The model under review builds one solid part; all positions refer to its coordinate system, in mm. Give positions to 0.01 mm unless a question says otherwise; leave off trailing zeros. Order: outer loops, then holes, each group sorted by start corner. A loop starts at its lowest first (then second) coordinate and runs counter-clockwise, first axis right, second up. Notation, with made-up numbers: (-2, -21.5) - (39, -21.5) arc R9 ccw to (39, -9.5) - close; hole circle Ø7 at (-39, 82). An arc over 180 degrees is marked (long way). Use CSV: the item, a comma, the result in double quotes. Start each with the question number.
```python
from build123d import *

# Parameters (mm, degrees)
SKETCH1_R           = 2.4892
BOSS_EXTRUDE1_DEPTH = 2.286


with BuildPart() as part:
    # Sketch1 → Boss-Extrude1 (new body)
    with BuildSketch(Plane.XY):
        with BuildLine():
            Line((459.749472964, 373.657281044), (426.729472964, 373.657281044))
            ThreePointArc((426.729472964, 373.657281044), (423.137370515, 375.145178596), (421.649472964, 378.737281044))
            Line((421.649472964, 378.737281044), (421.649472964, 387.627281044))
            ThreePointArc((421.649472964, 387.627281044), (423.137370515, 391.219383493), (426.729472964, 392.707281044))
            Line((426.729472964, 392.707281044), (537.219472964, 392.707281044))
            ThreePointArc((537.219472964, 392.707281044), (540.811575412, 391.219383493), (542.299472964, 387.627281044))
            Line((542.299472964, 387.627281044), (542.299472964, 277.137281044))
            ThreePointArc((542.299472964, 277.137281044), (540.811575412, 273.545178596), (537.219472964, 272.057281044))
            Line((537.219472964, 272.057281044), (528.329472964, 272.057281044))
            ThreePointArc((528.329472964, 272.057281044), (524.737370515, 273.545178596), (523.249472964, 277.137281044))
            Line((523.249472964, 277.137281044), (523.249472964, 310.157281044))
            ThreePointArc((523.249472964, 310.157281044), (504.650753569, 355.05856165), (459.749472964, 373.657281044))
        make_face()
        with Locations((431.174472964, 383.182281044)):
            Circle(SKETCH1_R, mode=Mode.SUBTRACT)
        with Locations((443.874472964, 383.182281044)):
            Circle(SKETCH1_R, mode=Mode.SUBTRACT)
        with Locations((456.574472964, 383.182281044)):
            Circle(SKETCH1_R, mode=Mode.SUBTRACT)
        with Locations((469.274472964, 383.182281044)):
            Circle(SKETCH1_R, mode=Mode.SUBTRACT)
        with Locations((481.974472964, 383.182281044)):
            Circle(SKETCH1_R, mode=Mode.SUBTRACT)
        with Locations((494.674472964, 383.182281044)):
            Circle(SKETCH1_R, mode=Mode.SUBTRACT)
        with Locations((507.374472964, 383.182281044)):
            Circle(SKETCH1_R, mode=Mode.SUBTRACT)
        with Locations((520.074472964, 383.182281044)):
            Circle(SKETCH1_R, mode=Mode.SUBTRACT)
        with Locations((532.774472964, 383.182281044)):
            Circle(SKETCH1_R, mode=Mode.SUBTRACT)
        with Locations((532.774472964, 370.482281044)):
            Circle(SKETCH1_R, mode=Mode.SUBTRACT)
        with Locations((532.774472964, 357.782281044)):
            Circle(SKETCH1_R, mode=Mode.SUBTRACT)
        with Locations((532.774472964, 345.082281044)):
            Circle(SKETCH1_R, mode=Mode.SUBTRACT)
        with Locations((532.774472964, 332.382281044)):
            Circle(SKETCH1_R, mode=Mode.SUBTRACT)
        with Locations((532.774472964, 319.682281044)):
            Circle(SKETCH1_R, mode=Mode.SUBTRACT)
        with Locations((532.774472964, 306.982281044)):
            Circle(SKETCH1_R, mode=Mode.SUBTRACT)
        with Locations((532.774472964, 294.282281044)):
            Circle(SKETCH1_R, mode=Mode.SUBTRACT)
        with Locations((532.774472964, 281.582281044)):
            Circle(SKETCH1_R, mode=Mode.SUBTRACT)
    extrude(amount=BOSS_EXTRUDE1_DEPTH)


solid = part.part
```
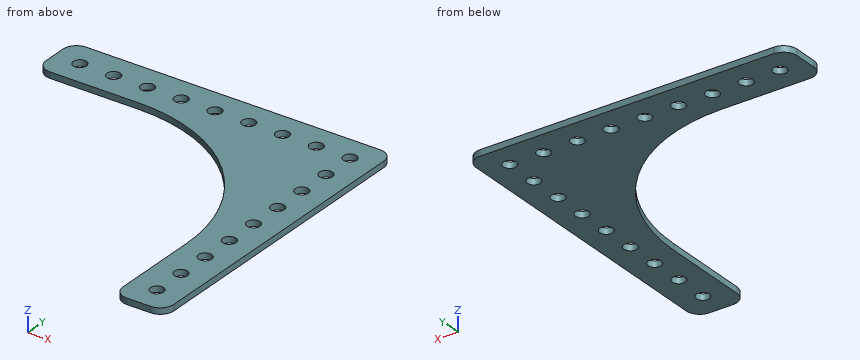
1. Consider section A-A (z = 1). State how many separate pieces and enclosed holes the cut face has, and give its area (3 significant figures).
2. Consider section B-B (x = 483). Give the boundary of the cut face in (y, z).
3. To check wall thickness, follow L1, parallel to X at y = 278, z = 1; L2, parallel to Y at x = 484, z = 1.7; L3, parallel to Y at x = 509, z = 2.15. State the ranges of each line that lie inside material, in increasing order. Write a range as [from, to].
4. Clearance check with flat-ended pins moving along their axes: pin 1 (6.5 mm diameter, centred on x = 532.77, y = 383.18, fed in from -Z); pin 2 (3 mm diameter, centred on x = 507.37, y = 383.18, fed in from -Z). State where each tip first meets the part, or that it passes through.
5. Consider section C-C (x = 470). Give the boundary of the cut face in (y, z).
6. Consider section D-D (y = 364). Give the boundary of the cut face in (x, z).
Answers follow:
1,separate pieces,"1"
1,enclosed holes,"17"
1,area,"4,740 mm^2"
2,outline,"(369.25, 0) - (380.91, 0) - (380.91, 2.29) - (369.25, 2.29) - close; (385.45, 0) - (392.71, 0) - (392.71, 2.29) - (385.45, 2.29) - close"
3,L1,"x = [523.25, 542.3]"
3,L2,"y = [368.84, 381.74], [384.63, 392.71]"
3,L3,"y = [350.24, 381.3], [385.07, 392.71]"
4,pin 1,"stops at z = 0"
4,pin 2,"passes through"
5,outline,"(372.82, 0) - (380.8, 0) - (380.8, 2.29) - (372.82, 2.29) - close; (385.56, 0) - (392.71, 0) - (392.71, 2.29) - (385.56, 2.29) - close"
6,outline,"(493.41, 0) - (542.3, 0) - (542.3, 2.29) - (493.41, 2.29) - close"
